For this review, take the finished solid that the model builds, in its own axes (mm). A direction names the side the tool comes from. Give positions to 0.01 mm unless a question says otherwise; leave off trailing zeros. Write each loop counter-clockwise with the first axis right and the second up, starting at its lowest first coordinate (ties: lowest second). Pieces come first, ordered by that corner, then holes. Notation, with made-up numbers: (40, 52.25) -> (57, 52.25) arc R26 ccw to (57, 66.25) -> close; hole circle Ø3 at (74, 43.25). An arc over 180 degrees is marked (long way). Return JSON: item names as keys, results as strings.
from build123d import *

# Parameters (mm, degrees)
F1_DEPTH  = 25
F3_D      = 2.5
F3_DEPTH  = 13.5
F3_TIP    = 0.7510757738
F4_W      = 21.9317121995
F4_H      = 25
F4_R      = 10
F4_W_2    = 1.5341439003
F5_DEPTH  = 10
F7_DEPTH  = 18.16
F8_SIZE2  = 2
F8_SIZE   = 5.5
F10_DEPTH = 14.7


with BuildPart() as f1:
    # F0 (on Top) → F1 (new body)
    with BuildSketch(Plane.XY):
        with BuildLine():
            ThreePointArc((10.9658560997, -6), (12.1103922572, -3.0965140685), (12.5, 0))
            ThreePointArc((12.5, 0), (12.1103922572, 3.0965140685), (10.9658560997, 6))
            Line((10.9658560997, 6), (-10.9658560997, 6))
            ThreePointArc((-10.9658560997, 6), (-12.5, 0), (-10.9658560997, -6))
            Line((-10.9658560997, -6), (10.9658560997, -6))
        make_face()
    extrude(amount=-F1_DEPTH)

    # F3
    with Locations(Plane.XY):
        with Locations((-8, 0), (8, 0)):
            Hole(F3_D / 2, depth=F3_DEPTH)
            with Locations((0, 0, -(F3_DEPTH + F3_TIP / 2))):  # 118° drill point
                Cone(0, F3_D / 2, F3_TIP, mode=Mode.SUBTRACT)

    # F4 (on face) → F5 (join)
    with BuildSketch(Plane.XZ.offset(6)):
        with Locations((0, -12.5)):
            Rectangle(F4_W, F4_H)
        with Locations((0, -12.5)):
            Circle(F4_R, mode=Mode.SUBTRACT)
        with Locations((-11.7329280499, -12.5)):
            Rectangle(F4_W_2, F4_H)
        with Locations((11.7329280499, -12.5)):
            Rectangle(F4_W_2, F4_H)
    extrude(amount=F5_DEPTH)

    # F6 (on face) → F7 (join)
    with BuildSketch(Plane(origin=(0, 0, -25), x_dir=(1, 0, 0), z_dir=(0, 0, -1))):
        with BuildLine():
            ThreePointArc((0, -6), (4.2426406871, -4.2426406871), (6, 0))
            ThreePointArc((6, 0), (-4.2426406871, 4.2426406871), (0, -6))
        make_face()
    extrude(amount=F7_DEPTH)

    # F8
    f8_edges = [f1.edges().sort_by_distance(p)[0] for p in [
        (0, -6, -43.16),
    ]]
    f8_side = f1.faces().sort_by_distance((0, 0, -43.16))[0]
    chamfer(f8_edges, length=F8_SIZE, length2=F8_SIZE2, reference=f8_side)

    # F9 (on face) → F10 (join)
    with BuildSketch(Plane.XY):
        Polygon((4.6187967668, -0.0070541219), (2.3155074321, 3.996468274), (-2.3032893346, 4.0035223959), (-4.6187967668, 0.0070541219), (-2.3155074321, -3.996468274), (2.3032893346, -4.0035223959), align=None)
    extrude(amount=F10_DEPTH)


solid = f1.part
1. Add section D-D, the plane z = -33.5. State the section outline as (x, y) points.
Results found:
{"outline": "circle Ø12 at (0, 0)"}
2. Add section B-B, the plane z = -12.5. State the section outline as (x, y) points.
Results found:
{"outline": "(-12.5, -16) -> (-10, -16) -> (-10, -6) -> (10, -6) -> (10, -16) -> (12.5, -16) -> (12.5, -6) -> (10.97, -6) arc R12.5 ccw to (10.97, 6) -> (-10.97, 6) arc R12.5 ccw to (-10.97, -6) -> (-12.5, -6) -> close; hole circle Ø2.5 at (-8, 0); hole circle Ø2.5 at (8, 0)"}
3. To check wall thickness, follow probe 1 along Y at (x, z) = (-8, -5.75); probe 2 along Z at (x, y) = (0, -7.75); probe 3 along Z at (x, y) = (-7.75, 4.25). State the ranges of each line that lie inside material, in increasing order.
Results found:
{"probe 1": "y = -16 to -1.25, 1.25 to 6", "probe 2": "z = -25 to -22.5, -2.5 to 0", "probe 3": "z = -25 to 0"}
4. For pin 1 (1.7 mm diameter, centred on x = 12, z = -10.5, fed in from +Y); pin 2 (3 mm diameter, centred on x = -8, y = 0, fed in from -Z); pin 3 (10 mm diameter, centred on x = -2.5, z = -11, fed in from -Y), all flat-tipped, find the tip position at first contact; note any pin that passes through.
Results found:
{"pin 1": "stops at y = 5.65", "pin 2": "stops at z = -25", "pin 3": "stops at y = -6"}
5. Add section C-C, the plane z = 1.5. State the section outline as (x, y) points.
Results found:
{"outline": "(-4.62, 0.01) -> (-2.32, -4) -> (2.3, -4) -> (4.62, -0.01) -> (2.32, 4) -> (-2.3, 4) -> close"}
6. The part is to be moulded in two halves that separate along X. For faces 1 (the flat face through (0, -6, -12)), 2 (the flat face through (3.48, 1.97, 7.25)), 3 (the flat face through (-3.445, 2.033, 7.247)), 4 (the flat face through (0, -5, 0)), say which applies: +X half, -X half, draft (parallel to the pull), parting line (faces both ways), or undercut.
Results found:
{"face 1": "undercut", "face 2": "+X half", "face 3": "-X half", "face 4": "draft"}
7. For faces 5 (the cylindrical face through (-7.94, -10.93, -18.58)), 6 (the cylindrical face through (9.25, 0.05, -6.84)), 7 (the flat face through (3.445, -2.033, 7.247)), 8 (the flat face through (-3.48, -1.97, 7.25)), list the 3-axis set-ups (+Z, -Z, +X, -X, +Y, -Y) from which the entire face can be reached by the end or side of a thin tool; tool diameter is ignored.
Results found:
{"face 5": "-Y", "face 6": "+Z", "face 7": "+Z, +X, -Y", "face 8": "+Z, -X, -Y"}
8. Add section A-A, the plane y = -13.75. State the section outline as (x, z) points.
Results found:
{"outline": "(-12.5, -25) -> (12.5, -25) -> (12.5, 0) -> (-12.5, 0) -> close; hole circle Ø20 at (0, -12.5)"}
